Study the drawing (mm; zero at the part's minimum x, y, z) and answer. A direction names the side the tool comes from. Coordinates: 2 decimals unless noted, no trailing zeros. Loops run counter-clockwise (first coordinate to the right, second up) from the corner with the lowest first, then second, coordinate; pieces in that order, holes last. Notation, with made-up numbers: (72, -37) -> (78, -37) arc R23 ccw to (78, -9) -> close; hole circle Ø8 at (59, -1). An arc over 180 degrees is marked (long way). One line per question, with ' | ' between items.
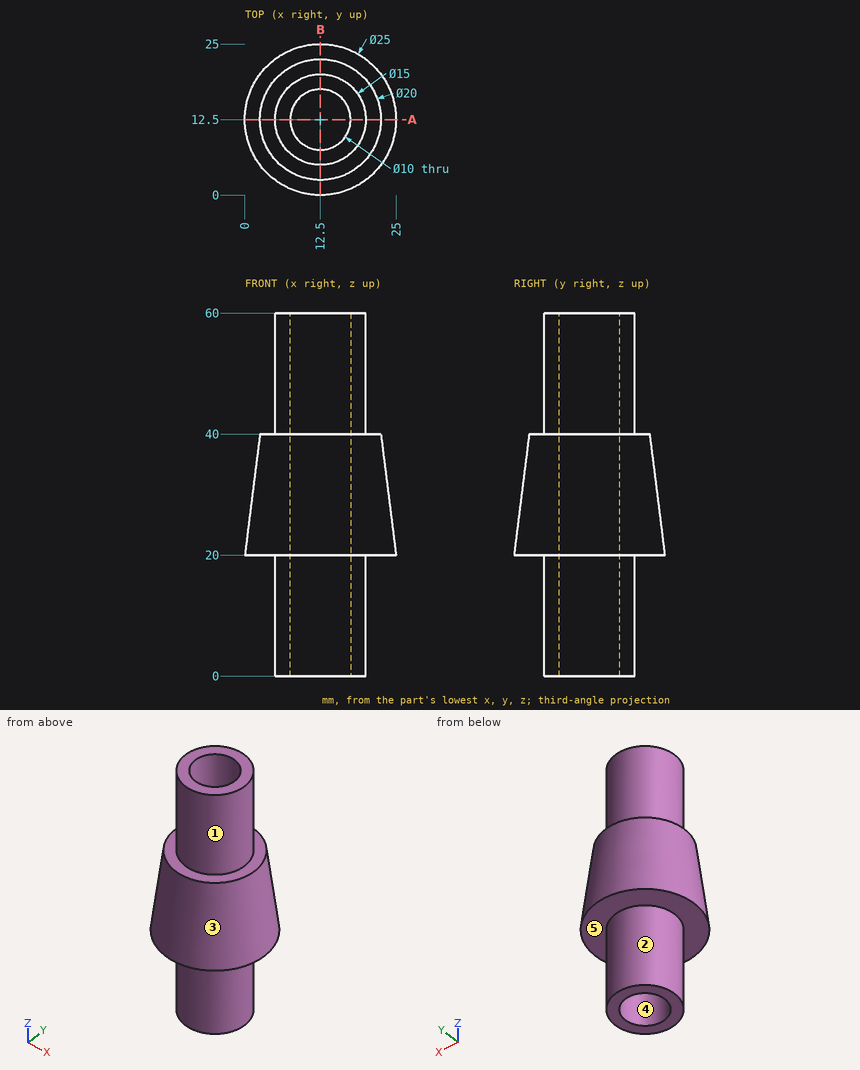
1) Find section A-A (y = 12.5). Write down the section's boundary in (x, z), plus the area to 3 significant figures.
Check values:
outline: (0, 20) -> (5, 20) -> (5, 0) -> (7.5, 0) -> (7.5, 60) -> (5, 60) -> (5, 40) -> (2.5, 40) -> close; (17.5, 0) -> (20, 0) -> (20, 20) -> (25, 20) -> (22.5, 40) -> (20, 40) -> (20, 60) -> (17.5, 60) -> close | area: 450 mm^2
2) For the marked faces 1 and 2, determine the directions among +Z, -Z, +X, -X, +Y, -Y from which every point of the face is accessible in a straight line to the end or side of a thin tool.
Check values:
face 1: +Z | face 2: -Z
3) The mould has two halves that part along X. Classify the marked faces 3, 4 and 5: released by +X, released by -X, zero draft, split by the parting line, or undercut.
Check values:
face 3: split by the parting line | face 4: undercut | face 5: zero draft
4) Find the intervals of material crossed by line 1 along X through (y, z) = (11, 50.5); line 2 along Y through (x, z) = (12.5, 25) (3 decimals); line 3 along Y through (x, z) = (15.75, 26.5), in increasing order.
Check values:
line 1: x = 5.15 to 7.73, 17.27 to 19.85 | line 2: y = 0.625 to 7.5, 17.5 to 24.375 | line 3: y = 1.27 to 8.7, 16.3 to 23.73
5) Flat-ended cylindrical pins translate along their axes: pin 1 (2 mm diameter, centred on x = 10, z = 34, fed in from -Y); pin 2 (6 mm diameter, centred on x = 7, y = 21.5, fed in from +Z); pin 3 (1.5 mm diameter, centred on x = 16.5, y = 3.5, fed in from -Z). Find the tip coordinate at first contact, or state that the pin passes through.
Check values:
pin 1: stops at y = 1.81 | pin 2: stops at z = 40 | pin 3: stops at z = 20
